```python
from build123d import *

# Parameters (mm, degrees)
BOSS_EXTRUDE1_DEPTH = 10
BOSS_EXTRUDE2_DEPTH = 2
SKETCH3_R           = 2
CUT_EXTRUDE1_DEPTH  = 4
CHAMFER1_SIZE       = 1.5


with BuildPart() as part:
    # Sketch1 → Boss-Extrude1 (new body)
    with BuildSketch(Plane.XY):
        Polygon((-25, 3.175), (-25, 7.175), (-5, 7.175), (-5, 12.175), (5, 12.175), (5, 7.175), (25, 7.175), (25, 3.175), (4, 3.175), (4, 0), (-4, 0), (-4, 3.175), align=None)
    extrude(amount=BOSS_EXTRUDE1_DEPTH)

    # Sketch2 → Boss-Extrude2 (add)
    with BuildSketch(Plane.XY.offset(10)):
        Polygon((-5, 12.175), (-25, 7.175), (-25, 3.175), (-4, 3.175), (-4, 0), (4, 0), (4, 3.175), (25, 3.175), (25, 7.175), (5, 12.175), align=None)
    extrude(amount=BOSS_EXTRUDE2_DEPTH)

    # Sketch3 → Cut-Extrude1 (cut)
    with BuildSketch(Plane(origin=(0, 7.175, 0), x_dir=(1, 0, 0), z_dir=(0, 1, 0))):
        with Locations((12, -5)):
            Circle(SKETCH3_R)
        with Locations((20, -5)):
            Circle(SKETCH3_R)
        with Locations((-12, -5)):
            Circle(SKETCH3_R)
        with Locations((-20, -5)):
            Circle(SKETCH3_R)
    extrude(amount=-CUT_EXTRUDE1_DEPTH, mode=Mode.SUBTRACT)

    # Chamfer1
    chamfer1_edges = [part.edges().sort_by_distance(p)[0] for p in [
        (4, 0, 6),
        (-4, 0, 6),
    ]]
    chamfer(chamfer1_edges, length=CHAMFER1_SIZE)


solid = part.part
```
Input: part model. Units: mm. Frame: model coordinates. A direction names the side the tool comes from. Round coordinates to 2 decimals unless told otherwise and drop trailing zeros. Loops run counter-clockwise (first coordinate to the right, second up) from the corner with the lowest first, then second, coordinate; pieces in that order, holes last. Notation, with made-up numbers: M 67,-14.5 L 72,-14.5 A28 ccw 72,21.5 Z; hole C 46,53 d7. An arc over 180 degrees is marked long. Answer in a Markdown table with one row per item. Add a question column.
1. Mould query, pull axis X, two halves, no side actions, for faces 1 (the face through (10.4, 5.2, 6.2)), 2 (the face through (5, 10, 5)), 3 (the face through (-14.9, 9.7, 11)). Classes: released by +X, released by -X, zero draft, split by the parting line, or undercut.
2. Section B-B (y = 8.25). Output: boundary loops of the cut face in (x, z).
3. Contact query for flat-ended pins moving along their axis: pin 1 (1.3 mm diameter, centred on y = 2, z = 3.5, fed in from -X); pin 2 (3.5 mm diameter, centred on x = 16, z = 8, fed in from -Y) (3 decimals); pin 3 (5.5 mm diameter, centred on x = -11.5, y = 8.5, fed in from -Z); pin 4 (4.5 mm diameter, centred on x = -20, z = 5, fed in from +Y) (3 decimals). Output: stop coordinate, or through.
4. Section D-D (x = 12). Output: boundary loops of the cut face in (y, z) (3 decimals), and give its area (3 significant figures).
5. Set-up query: faces 4 (the face through (4, 2, 6)), 5 (the face through (10, 9, 10)), 6 (the face through (-4, 2, 6)). Return all of +Z, -Z, +X, -X, +Y, -Y with unobstructed straight access to the full face (end or side cutting, diameter ignored); none if empty.
6. Section A-A (z = 5). Give the number of separate pieces and of enclosed holes in the cut face, and give its area (3 significant figures).
7. Section C-C (y = 6.25). Output: boundary loops of the cut face in (x, z), and give its area (3 significant figures).
8. Ray query, probe 1 along X at (y, z) = (5.25, 5); probe 2 along Z at (x, y) = (-20, 5); probe 3 along Y at (x, z) = (-12.5, 2) (3 decimals). Return the intervals inside material, ascending.
Values follow:
| question | item | result |
|---|---|---|
| 1 | face 1 | undercut |
| 1 | face 2 | released by +X |
| 1 | face 3 | released by -X |
| 2 | outline | M -20.7,10 L -5,10 L -5,0 L 5,0 L 5,10 L 20.7,10 L 20.7,12 L -20.7,12 Z |
| 3 | pin 1 | x = -4 |
| 3 | pin 2 | y = 3.175 |
| 3 | pin 3 | z = 0 |
| 3 | pin 4 | y = 7.175 |
| 4 | outline | M 3.175,0 L 7.175,0 L 7.175,3 L 3.175,3 Z; M 3.175,7 L 7.175,7 L 7.175,10 L 10.425,10 L 10.425,12 L 3.175,12 Z |
| 4 | area | 38.5 mm^2 |
| 5 | face 4 | +Z, -Z, +X, -Y |
| 5 | face 5 | -Z, +X, +Y |
| 5 | face 6 | +Z, -Z, -X, -Y |
| 6 | separate pieces | 5 |
| 6 | enclosed holes | 0 |
| 6 | area | 209 mm^2 |
| 7 | outline | M -25,0 L 25,0 L 25,12 L -25,12 Z; hole C -20,5 d4; hole C -12,5 d4; hole C 12,5 d4; hole C 20,5 d4 |
| 7 | area | 550 mm^2 |
| 8 | probe 1 | -25 to -22, -18 to -14, -10 to 10, 14 to 18, 22 to 25 |
| 8 | probe 2 | 0 to 3, 7 to 12 |
| 8 | probe 3 | 3.175 to 7.175 |
